Geometry: see drawing. Coordinates: mm, zero at the bounding-box minimum. A direction names the side the tool comes from. Coordinates: 2 decimals unless noted, no trailing zeros. Order: outer loops, then holes, each group sorted by start corner. A loop starts at its lowest first (then second) coordinate and runs counter-clockwise, first axis right, second up.
Item 1: Reachability of the marked faces 1 and 2 from +Z, -Z, +X, -X, +Y, -Y: full face, straight path, thin tool, end or side. Return the list, or none.
Item 2: Section B-B on y = 93.5. Return the cut outline in (x, z), then the cut area to 3 significant figures.
Item 3: Mould query, pull axis Y, two halves, no side actions, for the marked faces 3, 4 and 5. Classes: released by +Y, released by -Y, zero draft, split by the parting line, or undercut.
Item 4: Section C-C on x = 30. Return the cut outline in (y, z).
Item 5: Ray query, line 1 (X direction, y = 74.5, z = 5.75); line 2 (Y direction, x = 37.5, z = 6.75); line 3 (Y direction, x = 38, z = 3.5) (1 decimal). Return the intervals inside material, ascending.
Item 6: Section A-A on z = 13.5. Return the cut outline in (x, y).
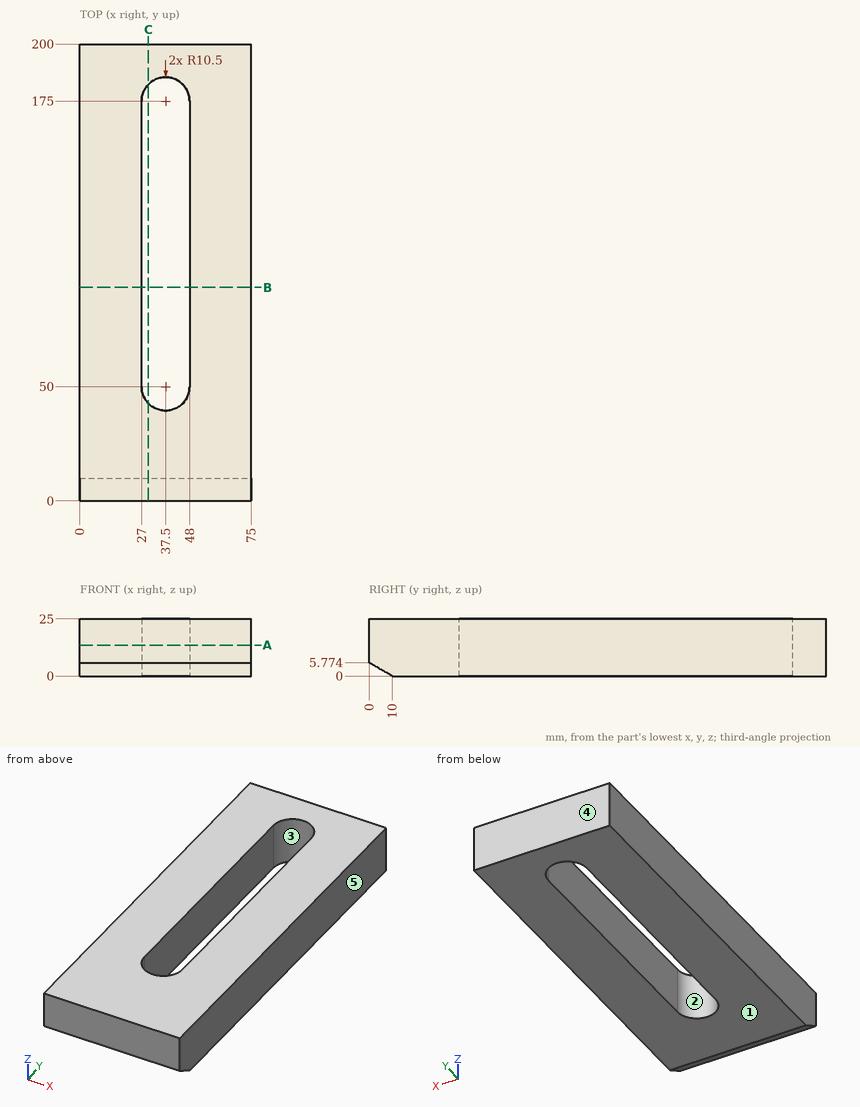
Answer list:
1. face 1: -Z, +X, -X, +Y, -Y
1. face 2: +Z, -Z
2. outline: (0, 0) - (27, 0) - (27, 25) - (0, 25) - close; (48, 0) - (75, 0) - (75, 25) - (48, 25) - close
2. area: 1,350 mm2
3. face 3: undercut
3. face 4: released by +Y
3. face 5: zero draft
4. outline: (0, 5.77) - (10, 0) - (42.65, 0) - (42.65, 25) - (0, 25) - close; (182.35, 0) - (200, 0) - (200, 25) - (182.35, 25) - close
5. line 1: x = 0 to 27, 48 to 75
5. line 2: y = 0 to 39.5, 185.5 to 200
5. line 3: y = 3.9 to 39.5, 185.5 to 200
6. outline: (0, 0) - (75, 0) - (75, 200) - (0, 200) - close; hole (27, 50) arc R10.5 ccw to (48, 50) - (48, 175) arc R10.5 ccw to (27, 175) - close
